The model under review builds one solid part; all positions refer to its coordinate system, in mm. Face numbers are marked on the shaded views. Coordinates: 2 decimals unless noted, no trailing zeros. Write each loop counter-clockwise with the first axis right and the second up, starting at its lowest first coordinate (ties: lowest second). Pieces come first, ordered by that corner, then holes.
1) For P1, Ø6, axis at x = 42.5, y = 6, coming from the -Z side; P2, Ø0.8, axis at y = -2, z = 22, coming from the +X side; P3, Ø2.5, axis at x = -41.5, y = 20, coming from the +Z side, all flat-tipped, find the tip position at first contact; note any pin that passes through.
2) For line 1 (X direction, y = 32.5, z = 9); line 2 (Y direction, x = -27, z = 20.5); line 3 (Y direction, x = -42.1, z = 0), list the stretches that pass through material, from the lowest coordinate up.
3) Mouldability with a two-part tool opening along X and no side actions: class the marked faces 1, 2 and 3 as released by +X, released by -X, zero draft, split by the parting line, or undercut.
4) Add section D-D, the plane z = -12. State the section outline as (x, y) points, then the cut area to 3 significant figures.
5) Add section A-A, the plane y = 7.5. State the section outline as (x, z) points.
6) Add section C-C, the plane z = -50.8. State the section outline as (x, y) points.
7) Add section B-B, the plane y = 22.4. State the section outline as (x, z) points, then the cut area to 3 significant figures.
from build123d import *

# Parameters (mm, degrees)
SKETCH1_R                     = 4.7625
BASE_FLANGE1_DEPTH            = 3
EDGE_FLANGE2_STRIP_W          = 13.4732
EDGE_FLANGE2_STRIP_H          = 3
EDGE_FLANGE2_STRIP_CUT_DEPTH  = 42.4
EDGE_FLANGE2_RELIEF_W         = 14.9732
EDGE_FLANGE2_RELIEF_H         = 1.5
EDGE_FLANGE2_RELIEF_CUT_DEPTH = 3
EDGE_FLANGE2_DEPTH            = 42.4
EDGE_FLANGE2_START            = 3
EDGE_FLANGE2_PROFILE_R        = 4.7625
EDGE_FLANGE2_FLAT_DEPTH       = 3
EDGE_FLANGE3_STRIP_W          = 13.4732
EDGE_FLANGE3_STRIP_H          = 3
EDGE_FLANGE3_STRIP_CUT_DEPTH  = 42.4
EDGE_FLANGE3_RELIEF_W         = 14.9732
EDGE_FLANGE3_RELIEF_H         = 1.5
EDGE_FLANGE3_RELIEF_CUT_DEPTH = 3
EDGE_FLANGE3_DEPTH            = 42.4
EDGE_FLANGE3_START            = 3
EDGE_FLANGE3_PROFILE_R        = 4.7625
EDGE_FLANGE3_FLAT_DEPTH       = 3


# Sheet-metal steps are written as plain solids
with BuildPart() as part:
    # Sketch1 → Base-Flange1 (new body)
    with BuildSketch(Plane(origin=(0, 0, 0), x_dir=(1, 0, 0), z_dir=(0, 1, 0))):
        with BuildLine():
            Line((-1.1, 76.2), (1.1, 76.2))
            ThreePointArc((1.1, 76.2), (29.384271247, 64.484271247), (41.1, 36.2))
            Line((41.1, 36.2), (41.1, -36.2))
            ThreePointArc((41.1, -36.2), (29.384271247, -64.484271247), (1.1, -76.2))
            Line((1.1, -76.2), (-1.1, -76.2))
            ThreePointArc((-1.1, -76.2), (-29.384271247, -64.484271247), (-41.1, -36.2))
            Line((-41.1, -36.2), (-41.1, 36.2))
            ThreePointArc((-41.1, 36.2), (-29.384271247, 64.484271247), (-1.1, 76.2))
        make_face()
        with Locations(Location((0, -50.8, 0), (0, 0, 270))):
            Circle(SKETCH1_R, mode=Mode.SUBTRACT)
        with Locations(Location((0, 50.8, 0), (0, 0, 90))):
            Circle(SKETCH1_R, mode=Mode.SUBTRACT)
    extrude(amount=-BASE_FLANGE1_DEPTH)

    # Edge-Flange2 strip (across the edge) → Edge-Flange2 strip cut (cut)
    with BuildSketch(Plane(origin=(41.1, 0, 21.2), x_dir=(-1, 0, 0), z_dir=(0, 0, -1))):
        with Locations((-6, -1.5)):
            Rectangle(EDGE_FLANGE2_STRIP_W, EDGE_FLANGE2_STRIP_H)
    extrude(amount=EDGE_FLANGE2_STRIP_CUT_DEPTH, mode=Mode.SUBTRACT)

    # Edge-Flange2 relief (on the sheet) → Edge-Flange2 relief cut (cut)
    with BuildSketch(Plane(origin=(40.3634, 0, 21.2), x_dir=(-1, 0, 0), z_dir=(0, 1, 0))):
        with Locations((-5.9866, 0.75)):
            Rectangle(EDGE_FLANGE2_RELIEF_W, EDGE_FLANGE2_RELIEF_H)
        with Locations((-5.9866, -43.15)):
            Rectangle(EDGE_FLANGE2_RELIEF_W, EDGE_FLANGE2_RELIEF_H)
    extrude(amount=-EDGE_FLANGE2_RELIEF_CUT_DEPTH, mode=Mode.SUBTRACT)

    # Edge-Flange2 bend section (across the edge) → Edge-Flange2 (add)
    with BuildSketch(Plane(origin=(41.1, 0, 21.2), x_dir=(-1, 0, 0), z_dir=(0, 0, -1))):
        with BuildLine():
            Line((-3, 0.7366), (0, 0.7366))
            ThreePointArc((0, 0.7366), (0.215745145, 0.215745145), (0.7366, 0))
            Line((0.7366, 0), (0.7366, -3))
            ThreePointArc((0.7366, -3), (-1.905575199, -1.905575199), (-3, 0.7366))
        make_face()
    extrude(amount=EDGE_FLANGE2_DEPTH)

    # Edge-Flange2 profile (on flange) → Edge-Flange2 flat (add)
    with BuildSketch(Plane(origin=(41.1, 0, 0), x_dir=(0, 0, -1), z_dir=(1, 0, 0)).offset(EDGE_FLANGE2_START)):
        with BuildLine():
            Line((-21.2, 27.8), (-21.2, 0.7366))
            Line((-21.2, 0.7366), (21.2, 0.7366))
            Line((21.2, 0.7366), (21.2, 27.8))
            ThreePointArc((21.2, 27.8), (15.342135624, 41.942135624), (1.2, 47.8))
            Line((1.2, 47.8), (-1.2, 47.8))
            ThreePointArc((-1.2, 47.8), (-15.342135624, 41.942135624), (-21.2, 27.8))
        make_face()
        with Locations((0, 22.4)):
            Circle(EDGE_FLANGE2_PROFILE_R, mode=Mode.SUBTRACT)
    extrude(amount=-EDGE_FLANGE2_FLAT_DEPTH)

    # Edge-Flange3 strip (across the edge) → Edge-Flange3 strip cut (cut)
    with BuildSketch(Plane(origin=(-41.1, 0, -21.2), x_dir=(1, 0, 0), z_dir=(0, 0, 1))):
        with Locations((-6, -1.5)):
            Rectangle(EDGE_FLANGE3_STRIP_W, EDGE_FLANGE3_STRIP_H)
    extrude(amount=EDGE_FLANGE3_STRIP_CUT_DEPTH, mode=Mode.SUBTRACT)

    # Edge-Flange3 relief (on the sheet) → Edge-Flange3 relief cut (cut)
    with BuildSketch(Plane(origin=(-40.3634, 0, -21.2), x_dir=(1, 0, 0), z_dir=(0, 1, 0))):
        with Locations((-5.9866, 0.75)):
            Rectangle(EDGE_FLANGE3_RELIEF_W, EDGE_FLANGE3_RELIEF_H)
        with Locations((-5.9866, -43.15)):
            Rectangle(EDGE_FLANGE3_RELIEF_W, EDGE_FLANGE3_RELIEF_H)
    extrude(amount=-EDGE_FLANGE3_RELIEF_CUT_DEPTH, mode=Mode.SUBTRACT)

    # Edge-Flange3 bend section (across the edge) → Edge-Flange3 (add)
    with BuildSketch(Plane(origin=(-41.1, 0, -21.2), x_dir=(1, 0, 0), z_dir=(0, 0, 1))):
        with BuildLine():
            Line((-3, 0.7366), (0, 0.7366))
            ThreePointArc((0, 0.7366), (0.215745145, 0.215745145), (0.7366, 0))
            Line((0.7366, 0), (0.7366, -3))
            ThreePointArc((0.7366, -3), (-1.905575199, -1.905575199), (-3, 0.7366))
        make_face()
    extrude(amount=EDGE_FLANGE3_DEPTH)

    # Edge-Flange3 profile (on flange) → Edge-Flange3 flat (add)
    with BuildSketch(Plane.ZY.offset(41.1).offset(EDGE_FLANGE3_START)):
        with BuildLine():
            Line((-21.2, 27.8), (-21.2, 0.7366))
            Line((-21.2, 0.7366), (21.2, 0.7366))
            Line((21.2, 0.7366), (21.2, 27.8))
            ThreePointArc((21.2, 27.8), (15.342135624, 41.942135624), (1.2, 47.8))
            Line((1.2, 47.8), (-1.2, 47.8))
            ThreePointArc((-1.2, 47.8), (-15.342135624, 41.942135624), (-21.2, 27.8))
        make_face()
        with Locations((0, 22.4)):
            Circle(EDGE_FLANGE3_PROFILE_R, mode=Mode.SUBTRACT)
    extrude(amount=-EDGE_FLANGE3_FLAT_DEPTH)


solid = part.part
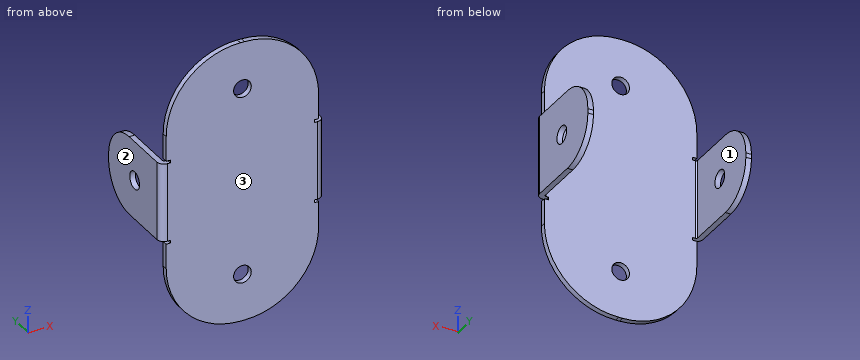
Geometry results:
1. P1: stops at z = -21.2
1. P2: stops at x = 38.86
1. P3: stops at z = 21.2
2. line 1: x = -44.1 to -41.1, 41.1 to 44.1
2. line 2: y = -3 to 0
2. line 3: y = -2.57 to 17.64, 27.16 to 47.8
3. face 1: undercut
3. face 2: released by -X
3. face 3: zero draft
4. outline: (-44.1, 0.74) arc R3.74 ccw to (-40.36, -3) - (40.36, -3) arc R3.74 ccw to (44.1, 0.74) - (44.1, 44.63) - (41.1, 44.63) - (41.1, 0.74) arc R0.74 cw to (40.36, 0) - (-40.36, 0) arc R0.74 cw to (-41.1, 0.74) - (-41.1, 44.63) - (-44.1, 44.63) - close
4. area: 527 mm2
5. outline: (-44.1, -21.2) - (-41.1, -21.2) - (-41.1, 21.2) - (-44.1, 21.2) - close; (41.1, -21.2) - (44.1, -21.2) - (44.1, 21.2) - (41.1, 21.2) - close
6. outline: (-38.34, -3) - (-4.76, -3) - (-4.76, 0) - (-38.34, 0) - close; (4.76, -3) - (38.34, -3) - (38.34, 0) - (4.76, 0) - close
7. outline: (-44.1, -21.2) - (-41.1, -21.2) - (-41.1, -4.76) - (-44.1, -4.76) - close; (-44.1, 4.76) - (-41.1, 4.76) - (-41.1, 21.2) - (-44.1, 21.2) - close; (41.1, -21.2) - (44.1, -21.2) - (44.1, -4.76) - (41.1, -4.76) - close; (41.1, 4.76) - (44.1, 4.76) - (44.1, 21.2) - (41.1, 21.2) - close
7. area: 197 mm2
